```python
from build123d import *

# Parameters (mm, degrees)
SKETCH1_W           = 30
SKETCH1_H           = 50
BOSS_EXTRUDE1_DEPTH = 1.5
SKETCH2_R           = 3.175
SKETCH2_R_2         = 1.6
CUT_EXTRUDE1_DEPTH  = 3
SKETCH3_W           = 3
SKETCH3_H           = 40
BOSS_EXTRUDE2_DEPTH = 10


with BuildPart() as part:
    # Sketch1 → Boss-Extrude1 (new body, symmetric)
    with BuildSketch(Plane(origin=(0, 0, 0), x_dir=(1, 0, 0), z_dir=(0, 1, 0))):
        Rectangle(SKETCH1_W, SKETCH1_H)
    extrude(amount=BOSS_EXTRUDE1_DEPTH, both=True)

    # Sketch2 → Cut-Extrude1 (cut)
    with BuildSketch(Plane(origin=(0, 1.5, 0), x_dir=(1, 0, 0), z_dir=(0, 1, 0))):
        Circle(SKETCH2_R)
        with Locations((0, 12)):
            Circle(SKETCH2_R_2)
    extrude(amount=-CUT_EXTRUDE1_DEPTH, mode=Mode.SUBTRACT)

    # Sketch3 → Boss-Extrude2 (add)
    with BuildSketch(Plane(origin=(0, 1.5, 0), x_dir=(1, 0, 0), z_dir=(0, 1, 0))):
        with Locations((11.5, 0)):
            Rectangle(SKETCH3_W, SKETCH3_H)
    boss_extrude2 = extrude(amount=BOSS_EXTRUDE2_DEPTH)

    # Mirror1: Boss-Extrude2 across plane
    add(boss_extrude2.mirror(Plane(origin=(0, 0, 0), x_dir=(0, 0, 1), z_dir=(1, 0, 0))))


solid = part.part
```
Source: CAD feature listing. Evaluate the final solid. Frame: model axes, mm. A direction names the side the tool comes from. Round coordinates to 2 decimals unless told otherwise and drop trailing zeros. Order: outer loops, then holes, each group sorted by start corner. A loop starts at its lowest first (then second) coordinate and runs counter-clockwise, first axis right, second up. Notation, with made-up numbers: (87, 45) -> (127, 45) arc R18 cw to (127, 53) -> close; hole circle Ø9 at (4.5, 77.5). An arc over 180 degrees is marked (long way). Use CSV: the item, a comma, the result in double quotes.
(1) Section A-A on y = 5.5. Return the cut outline in (x, z).
Report:
outline,"(-13, -20) -> (-10, -20) -> (-10, 20) -> (-13, 20) -> close; (10, -20) -> (13, -20) -> (13, 20) -> (10, 20) -> close"
(2) Section C-C on x = 0. Return the cut outline in (y, z) (3 decimals).
Report:
outline,"(-1.5, -25) -> (1.5, -25) -> (1.5, -13.6) -> (-1.5, -13.6) -> close; (-1.5, -10.4) -> (1.5, -10.4) -> (1.5, -3.175) -> (-1.5, -3.175) -> close; (-1.5, 3.175) -> (1.5, 3.175) -> (1.5, 25) -> (-1.5, 25) -> close"
(3) Section B-B on z = -12. Return the cut outline in (x, y).
Report:
outline,"(-15, -1.5) -> (-1.6, -1.5) -> (-1.6, 1.5) -> (-10, 1.5) -> (-10, 11.5) -> (-13, 11.5) -> (-13, 1.5) -> (-15, 1.5) -> close; (1.6, -1.5) -> (15, -1.5) -> (15, 1.5) -> (13, 1.5) -> (13, 11.5) -> (10, 11.5) -> (10, 1.5) -> (1.6, 1.5) -> close"
(4) Access query for faces 1 (the face through (-11, 6, -20)), 2 (the face through (11, 6, 20)), 3 (the face through (-10, 6, 0)). Directions: +Z, -Z, +X, -X, +Y, -Y. A direction counts if a zero-diameter tool reaches every point of the face in a straight line with its end or side. Return the directions, or none.
Report:
face 1,"-Z, +X, -X, +Y"
face 2,"+Z, +X, -X, +Y"
face 3,"+Z, -Z, +Y"
(5) Pull-direction query (X, two-part tool) for faces 4 (the face through (10, 6, 0)), 5 (the face through (15, 0, 0)), 6 (the face through (11, 6, -20)); classes: +X half, -X half, draft (parallel to the pull), parting line (faces both ways), or undercut.
Report:
face 4,"undercut"
face 5,"+X half"
face 6,"draft"
(6) Ray query, L1, parallel to Z at x = 0, y = -0.45 (3 decimals); L2, parallel to X at y = 6.5, z = -11.5; L3, parallel to X at y = 0, z = -12. Return the intervals inside material, ascending.
Report:
L1,"-25 to -13.6, -10.4 to -3.175, 3.175 to 25"
L2,"-13 to -10, 10 to 13"
L3,"-15 to -1.6, 1.6 to 15"
(7) Section D-D on y = 0.25. Return the cut outline in (x, z) (3 decimals).
Report:
outline,"(-15, -25) -> (15, -25) -> (15, 25) -> (-15, 25) -> close; hole circle Ø6.35 at (0, 0); hole circle Ø3.2 at (0, -12)"
(8) First-contact query: pin 1 Ø3.5 at (x, y) = (-12, 6) entering from +Z; pin 2 Ø3 at (y, z) = (7, 3) entering from -X; pin 3 Ø5 at (y, z) = (4.5, 8.5) entering from +X. Flat tips, straight axial feed; report the tip coordinate or a pass-through.
Report:
pin 1,"z = 20"
pin 2,"x = -13"
pin 3,"x = 13"
